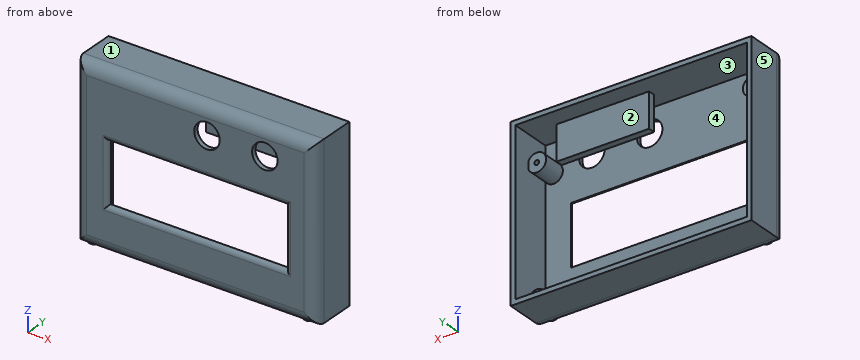
```python
from build123d import *

# Parameters (mm, degrees)
SKETCH1_W           = 104
SKETCH1_H           = 74
SKETCH1_W_2         = 100
SKETCH1_H_2         = 70
BOSS_EXTRUDE2_DEPTH = 20
SKETCH1_3_W         = 100
SKETCH1_3_H         = 70
SKETCH1_3_R         = 5.5
SKETCH1_3_W_2       = 77
SKETCH1_3_H_2       = 26
BOSS_EXTRUDE3_DEPTH = 2
FILLET1_R           = 5
FILLET2_R           = 2
SKETCH3_R           = 4
SKETCH3_R_2         = 1
BOSS_EXTRUDE4_DEPTH = 10
SKETCH4_W           = 40
SKETCH4_H           = 3
BOSS_EXTRUDE5_DEPTH = 15


with BuildPart() as part:
    # Sketch1 → Boss-Extrude2 (new body)
    with BuildSketch(Plane(origin=(0, 0, 0), x_dir=(1, 0, 0), z_dir=(0, 1, 0))):
        with Locations((-31.943816067, -36.302599947)):
            Rectangle(SKETCH1_W, SKETCH1_H)
        with Locations((-31.943816067, -36.302599947)):
            Rectangle(SKETCH1_W_2, SKETCH1_H_2, mode=Mode.SUBTRACT)
    extrude(amount=BOSS_EXTRUDE2_DEPTH)

    # Sketch1<3> → Boss-Extrude3 (add)
    with BuildSketch(Plane(origin=(0, 0, 0), x_dir=(1, 0, 0), z_dir=(0, 1, 0))):
        with Locations((-31.943816067, -36.302599947)):
            Rectangle(SKETCH1_3_W, SKETCH1_3_H)
        with Locations(Location((-1.943816067, -61.302599947, 0), (0, 0, 270))):
            Circle(SKETCH1_3_R, mode=Mode.SUBTRACT)
        with Locations(Location((-26.943816067, -61.302599947, 0), (0, 0, 270))):
            Circle(SKETCH1_3_R, mode=Mode.SUBTRACT)
        with Locations((-31.443816067, -31.602599947)):
            Rectangle(SKETCH1_3_W_2, SKETCH1_3_H_2, mode=Mode.SUBTRACT)
    extrude(amount=BOSS_EXTRUDE3_DEPTH)

    # Fillet1
    fillet1_edges = [part.edges().sort_by_distance(p)[0] for p in [
        (-83.943816067, 0, 36.302599947),
        (-31.943816067, 0, 73.302599947),
        (20.056183933, 0, 36.302599947),
        (-31.943816067, 0, -0.697400053),
    ]]
    fillet(fillet1_edges, radius=FILLET1_R)

    # Fillet2
    fillet2_edges = [part.edges().sort_by_distance(p)[0] for p in [
        (-69.943816067, 0, 31.602599947),
        (-31.443816067, 0, 44.602599947),
        (7.056183933, 0, 31.602599947),
        (-31.443816067, 0, 18.602599947),
    ]]
    fillet(fillet2_edges, radius=FILLET2_R - 0.0001)  # a hair under: the kernel refuses the full size

    # Sketch3 → Boss-Extrude4 (add)
    # profile 1 of 4: a face of its own
    with BuildSketch(Plane(origin=(0, 2, 0), x_dir=(1, 0, 0), z_dir=(0, 1, 0))):
        with Locations((-78.443816067, -3.802599947)):
            Circle(SKETCH3_R)
        with Locations(Location((-78.443816067, -3.802599947, 0), (0, 0, 270))):
            Circle(SKETCH3_R_2, mode=Mode.SUBTRACT)
    # profile 2 of 4: a face of its own
    with BuildSketch(Plane(origin=(0, 2, 0), x_dir=(1, 0, 0), z_dir=(0, 1, 0))):
        with Locations((14.556183933, -3.802599947)):
            Circle(SKETCH3_R)
        with Locations(Location((14.556183933, -3.802599947, 0), (0, 0, 270))):
            Circle(SKETCH3_R_2, mode=Mode.SUBTRACT)
    # profile 3 of 4: a face of its own
    with BuildSketch(Plane(origin=(0, 2, 0), x_dir=(1, 0, 0), z_dir=(0, 1, 0))):
        with Locations((-78.443816067, -58.802599947)):
            Circle(SKETCH3_R)
        with Locations(Location((-78.443816067, -58.802599947, 0), (0, 0, 270))):
            Circle(SKETCH3_R_2, mode=Mode.SUBTRACT)
    # profile 4 of 4: a face of its own
    with BuildSketch(Plane(origin=(0, 2, 0), x_dir=(1, 0, 0), z_dir=(0, 1, 0))):
        with Locations((14.556183933, -58.802599947)):
            Circle(SKETCH3_R)
        with Locations(Location((14.556183933, -58.802599947, 0), (0, 0, 270))):
            Circle(SKETCH3_R_2, mode=Mode.SUBTRACT)
    extrude(amount=BOSS_EXTRUDE4_DEPTH)

    # Sketch4 → Boss-Extrude5 (add)
    with BuildSketch(Plane(origin=(0, 0, 71.302599947), x_dir=(-1, 0, 0), z_dir=(0, 0, -1))):
        with Locations((13.943816067, 10.5)):
            Rectangle(SKETCH4_W, SKETCH4_H)
    extrude(amount=BOSS_EXTRUDE5_DEPTH)


solid = part.part
```
The listing builds one solid part. Answer for the finished solid, in the listing's coordinates (mm). Face numbers are marked on the shaded views. A direction names the side the tool comes from. Round coordinates to 2 decimals unless told otherwise and drop trailing zeros. Loops run counter-clockwise (first coordinate to the right, second up) from the corner with the lowest first, then second, coordinate; pieces in that order, holes last.
1) A cutting plane is placed at D-D on z = 51.5. Determine the outline of the cut face in (x, y).
Outcome:
outline: (-83.94, 5) arc R5 ccw to (-78.94, 0) - (15.06, 0) arc R5 ccw to (20.06, 5) - (20.06, 20) - (18.06, 20) - (18.06, 2) - (-81.94, 2) - (-81.94, 20) - (-83.94, 20) - close
2) Consider line 1 (X direction, y = 13.25, z = 36); line 2 (Z direction, x = -17, y = 14.5); line 3 (Z direction, x = -20.5, y = 10.5). Determine where each line is inside the solid, lowest interval first.
Outcome:
line 1: x = -83.94 to -81.94, 18.06 to 20.06
line 2: z = -0.7 to 1.3, 71.3 to 73.3
line 3: z = -0.7 to 1.3, 56.3 to 73.3
3) A cutting plane is placed at C-C on y = 17.5. Determine the outline of the cut face in (x, z).
Outcome:
outline: (-83.94, -0.7) - (20.06, -0.7) - (20.06, 73.3) - (-83.94, 73.3) - close; hole (-81.94, 1.3) - (18.06, 1.3) - (18.06, 71.3) - (-81.94, 71.3) - close
4) Given P1, Ø3.5, axis at x = -79, z = 6, coming from the +Y side; P2, Ø1.2, axis at x = 14.56, z = 58.8, coming from the +Y side; P3, Ø9, axis at x = -26.94, z = 61.3, coming from the -Y side, each flat-ended and moving along its own axis, determine where each tip first touches the part or whether it passes through.
Outcome:
P1: stops at y = 12
P2: stops at y = 2
P3: stops at y = 9
5) For the marked faces 4 and 5, determine the directions among +Z, -Z, +X, -X, +Y, -Y from which every point of the face is accessible in a straight line to the end or side of a thin tool.
Outcome:
face 4: none
face 5: +Z, -Z, -X, +Y, -Y
6) For a pull along Y with two mould halves and no side action, classify the marked faces 1, 2 and 3 as released by +Y, released by -Y, zero draft, split by the parting line, or undercut.
Outcome:
face 1: zero draft
face 2: released by +Y
face 3: undercut
